from build123d import *

# Parameters (mm, degrees)
BOSS_EXTRUDE1_DEPTH = 18
SKETCH2_R           = 2.35
CUT_EXTRUDE1_DEPTH  = 18
SKETCH4_W           = 1.5
SKETCH4_H           = 6
BOSS_EXTRUDE3_DEPTH = 2
BOSS_EXTRUDE2_DEPTH = 3


with BuildPart() as part:
    # Sketch1 → Boss-Extrude1 (new body)
    with BuildSketch(Plane.XY):
        Polygon((0, 0), (-38, 0), (-38, 5), (-5, 5), (-5, 38), (0, 38), align=None)
    extrude(amount=BOSS_EXTRUDE1_DEPTH)

    # Sketch2 → Cut-Extrude1 (cut)
    with BuildSketch(Plane(origin=(0, 5, 0), x_dir=(1, 0, 0), z_dir=(0, 1, 0))):
        with Locations((-30, -9)):
            Circle(SKETCH2_R)
        with Locations((-15, -9)):
            Circle(SKETCH2_R)
    cut_extrude1 = extrude(amount=-CUT_EXTRUDE1_DEPTH, mode=Mode.SUBTRACT)

    # Sketch4 → Boss-Extrude3 (add)
    with BuildSketch(Plane.XZ):
        with Locations((-37.25, 9)):
            Rectangle(SKETCH4_W, SKETCH4_H)
        with Locations((-8, 9)):
            Rectangle(SKETCH4_W, SKETCH4_H)
    boss_extrude3 = extrude(amount=BOSS_EXTRUDE3_DEPTH)

    # Mirror1: Cut-Extrude1, Boss-Extrude3 across plane
    add(cut_extrude1.mirror(Plane(origin=(0, 0, 0), x_dir=(0, 0, 1), z_dir=(0.707106781, 0.707106781, 0))), mode=Mode.SUBTRACT)
    add(boss_extrude3.mirror(Plane(origin=(0, 0, 0), x_dir=(0, 0, 1), z_dir=(0.707106781, 0.707106781, 0))))

    # Sketch3 → Boss-Extrude2 (add)
    with BuildSketch(Plane(origin=(0, 0, 0), x_dir=(-1, 0, 0), z_dir=(0, 0, -1))):
        Polygon((5, 38), (38, 5), (5, 5), align=None)
    extrude(amount=-BOSS_EXTRUDE2_DEPTH)


solid = part.part
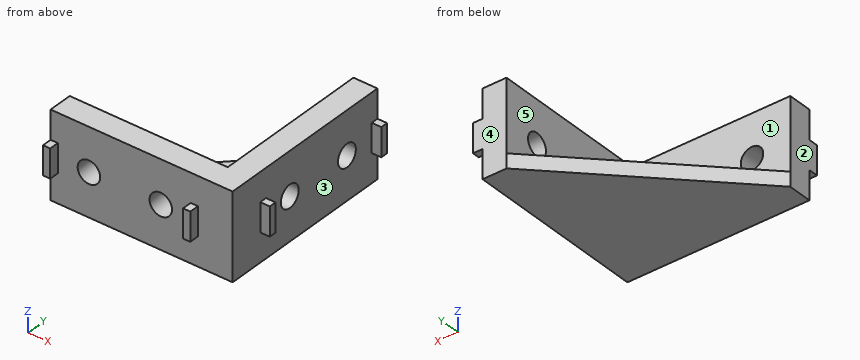
Part model, mm, in its own coordinate system. Face numbers are marked on the shaded views. A direction names the side the tool comes from. Round coordinates to 2 decimals unless told otherwise and drop trailing zeros. Write each loop counter-clockwise with the first axis right and the second up, starting at its lowest first coordinate (ties: lowest second). Pieces come first, ordered by that corner, then holes. Notation, with made-up numbers: (12.25, 67) - (24.25, 67) arc R33 cw to (24.25, 105) - close; hole circle Ø4 at (25, -33). An arc over 180 degrees is marked (long way). Use CSV: the item, a comma, the result in double quotes.
Item 1: Slice it at C-C, the plane x = -30. Write the cut outline in (y, z).
Results list:
outline,"(0, 0) - (13, 0) - (13, 3) - (5, 3) - (5, 6.65) - (0, 6.65) - close; (0, 11.35) - (5, 11.35) - (5, 18) - (0, 18) - close"
Item 2: Wall check: L1, parallel to Y at x = -2.4, z = 9; L2, parallel to X at y = 3.4, z = 9; L3, parallel to Z at x = -30, y = 1.85. Give the ranges that are in metal, low to high.
Results list:
L1,"y = 0 to 12.65, 17.35 to 27.65, 32.35 to 38"
L2,"x = -38 to -32.35, -27.65 to -17.35, -12.65 to 0"
L3,"z = 0 to 6.65, 11.35 to 18"
Item 3: Slice it at D-D, the plane y = 2. Write the cut outline in (x, z).
Results list:
outline,"(-38, 0) - (0, 0) - (0, 18) - (-38, 18) - close; hole circle Ø4.7 at (-30, 9); hole circle Ø4.7 at (-15, 9)"
Item 4: Slice it at B-B, the plane z = 9. Count the separate pieces of the cut face and the enclosed holes in it, then the cut area to 3 significant figures.
Results list:
separate pieces,"5"
enclosed holes,"0"
area,"273 mm²"
Item 5: Pull direction Y, two halves, no side cores. Call the marked faces 3, 4 and 5: pulls with the +Y half, pulls with the -Y half, needs draft (parallel to the pull), parting line crosses it, or undercut.
Results list:
face 3,"undercut"
face 4,"pulls with the +Y half"
face 5,"needs draft"
Item 6: Flat gauge pins, fed straight in: P1, Ø16.5, axis at x = -24, y = 26.5, coming from the +Z side; P2, Ø5, axis at y = 16.5, z = 12.5, coming from the +X side; P3, Ø1.2, axis at x = -8, y = -1, coming from the -Z side. Where does each tip first touch, or does it go through?
Results list:
P1,"stops at z = 3"
P2,"stops at x = 0"
P3,"stops at z = 6"
Item 7: Tool access for the marked faces 1 and 2: list every direction of +Z, -Z, +X, -X, +Y, -Y with a clear straight run to the whole face (end or side of a thin tool).
Results list:
face 1,"+Z, -X, +Y"
face 2,"+Z, -Z, -X, +Y, -Y"
Item 8: Slice it at A-A, the plane y = 30. Write the cut outline in (x, z), then the cut area to 3 significant figures.
Results list:
outline,"(-13, 0) - (0, 0) - (0, 6.65) - (-5, 6.65) - (-5, 3) - (-13, 3) - close; (-5, 11.35) - (0, 11.35) - (0, 18) - (-5, 18) - close"
area,"90.5 mm²"
